Geometry: final body of the model. Coordinates: model frame, mm. A direction names the side the tool comes from. Round coordinates to 2 decimals unless told otherwise and drop trailing zeros. Loops run counter-clockwise (first coordinate to the right, second up) from the corner with the lowest first, then second, coordinate; pieces in that order, holes last. Notation, with made-up numbers: M 40.25,51.25 L 89.25,51.25 A23 ccw 89.25,74.25 Z; hole C -21.5,26 d8. An arc over 180 degrees is marked long. Write each question's results on one line, items separated by ' | '.
```python
from build123d import *

# Parameters (mm, degrees)
BOX018_W               = 0.3
BOX018_H               = 3.5
BOX018_DEPTH           = 4
BOX018_PLACEMENT_ANGLE = 120
BOX017_W               = 0.3
BOX017_H               = 3.5
BOX017_DEPTH           = 4
BOX017_PLACEMENT_ANGLE = 120
BOX016_W               = 0.3
BOX016_H               = 3.5
BOX016_DEPTH           = 4
BOX016_PLACEMENT_ANGLE = 120
BOX014_W               = 0.3
BOX014_H               = 3.5
BOX014_DEPTH           = 4
BOX003_W               = 0.3
BOX003_H               = 3.5
BOX003_DEPTH           = 4
BOX003_PLACEMENT_ANGLE = 30
BOX001_W               = 0.3
BOX001_H               = 3.5
BOX001_DEPTH           = 4
BOX001_PLACEMENT_ANGLE = 30
BOX002_W               = 0.3
BOX002_H               = 3.5
BOX002_DEPTH           = 4
BOX015_W               = 0.3
BOX015_H               = 3.5
BOX015_DEPTH           = 4
BOX004_W               = 0.3
BOX004_H               = 3.5
BOX004_DEPTH           = 4
BOX_W                  = 8
BOX_H                  = 4
BOX_DEPTH              = 4
CYLINDER001_R          = 2
CYLINDER001_DEPTH      = 4
CYLINDER_R             = 2
CYLINDER_DEPTH         = 4


with BuildPart() as cube018:
    # Box018 → Box018 (new body)
    with BuildSketch(Plane.XY):
        with Locations((0.15, 1.75)):
            Rectangle(BOX018_W, BOX018_H)
    extrude(amount=BOX018_DEPTH)


with BuildPart() as cube018_1:
    # Box018 placement: moved
    add(cube018.part.moved(Location((7.892915, 0.015358, 0))).rotate(Axis((7.892915, 0.015358, 0), (0, 0, -1)), BOX018_PLACEMENT_ANGLE))


with BuildPart() as cube017:
    # Box017 → Box017 (new body)
    with BuildSketch(Plane.XY):
        with Locations((0.15, 1.75)):
            Rectangle(BOX017_W, BOX017_H)
    extrude(amount=BOX017_DEPTH)


with BuildPart() as cube017_1:
    # Box017 placement: moved
    add(cube017.part.moved(Location((10.852236, 1.891667, 0))).rotate(Axis((10.852236, 1.891667, 0), (0, 0, 1)), BOX017_PLACEMENT_ANGLE))


with BuildPart() as cube016:
    # Box016 → Box016 (new body)
    with BuildSketch(Plane.XY):
        with Locations((0.15, 1.75)):
            Rectangle(BOX016_W, BOX016_H)
    extrude(amount=BOX016_DEPTH)


with BuildPart() as cube016_1:
    # Box016 placement: moved
    add(cube016.part.moved(Location((-0.004428, -0.104039, 0))).rotate(Axis((-0.004428, -0.104039, 0), (0, 0, 1)), BOX016_PLACEMENT_ANGLE))


with BuildPart() as cube014:
    # Box014 → Box014 (new body)
    with BuildSketch(Plane(origin=(2.3, 0, 0), x_dir=(1, 0, 0), z_dir=(0, 0, 1))):
        with Locations((0.15, 1.75)):
            Rectangle(BOX014_W, BOX014_H)
    extrude(amount=BOX014_DEPTH)


with BuildPart() as cube003:
    # Box003 → Box003 (new body)
    with BuildSketch(Plane.XY):
        with Locations((0.15, 1.75)):
            Rectangle(BOX003_W, BOX003_H)
    extrude(amount=BOX003_DEPTH)


with BuildPart() as cube003_1:
    # Box003 placement: moved
    add(cube003.part.moved(Location((7.7321, -3, 0))).rotate(Axis((7.7321, -3, 0), (0, 0, 1)), BOX003_PLACEMENT_ANGLE))


with BuildPart() as cube001:
    # Box001 → Box001 (new body)
    with BuildSketch(Plane.XY):
        with Locations((0.15, 1.75)):
            Rectangle(BOX001_W, BOX001_H)
    extrude(amount=BOX001_DEPTH)


with BuildPart() as cube001_1:
    # Box001 placement: moved
    add(cube001.part.rotate(Axis((0, 0, 0), (0, 0, 1)), BOX001_PLACEMENT_ANGLE))


with BuildPart() as cube002:
    # Box002 → Box002 (new body)
    with BuildSketch(Plane(origin=(6, 0, 0), x_dir=(1, 0, 0), z_dir=(0, 0, 1))):
        with Locations((0.15, 1.75)):
            Rectangle(BOX002_W, BOX002_H)
    extrude(amount=BOX002_DEPTH)


with BuildPart() as cube015:
    # Box015 → Box015 (new body)
    with BuildSketch(Plane(origin=(3.6, -3.5, 0), x_dir=(1, 0, 0), z_dir=(0, 0, 1))):
        with Locations((0.15, 1.75)):
            Rectangle(BOX015_W, BOX015_H)
    extrude(amount=BOX015_DEPTH)


with BuildPart() as fusion008:
    # Box004 → Box004 (new body)
    with BuildSketch(Plane(origin=(0, -3.5, 0), x_dir=(1, 0, 0), z_dir=(0, 0, 1))):
        with Locations((0.15, 1.75)):
            Rectangle(BOX004_W, BOX004_H)
    extrude(amount=BOX004_DEPTH)

    # Fusion008: union Cube018, Cube017, Cube016, Cube014, Cube003, Cube001, Cube002, Cube015
    add(cube018_1.part)
    add(cube017_1.part)
    add(cube016_1.part)
    add(cube014.part)
    add(cube003_1.part)
    add(cube001_1.part)
    add(cube002.part)
    add(cube015.part)


with BuildPart() as cube:
    # Box → Box (new body)
    with BuildSketch(Plane(origin=(0, -2, 0), x_dir=(1, 0, 0), z_dir=(0, 0, 1))):
        with Locations((4, 2)):
            Rectangle(BOX_W, BOX_H)
    extrude(amount=BOX_DEPTH)


with BuildPart() as cylinder001:
    # Cylinder001 → Cylinder001 (new body)
    with BuildSketch(Plane(origin=(8, 0, 0), x_dir=(1, 0, 0), z_dir=(0, 0, 1))):
        Circle(CYLINDER001_R)
    extrude(amount=CYLINDER001_DEPTH)


with BuildPart() as fusion014:
    # Cylinder → Cylinder (new body)
    with BuildSketch(Plane.XY):
        Circle(CYLINDER_R)
    extrude(amount=CYLINDER_DEPTH)

    # Fusion: union Cube, Cylinder001
    add(cube.part)
    add(cylinder001.part)

    # Fusion014: union Fusion008
    add(fusion008.part)


solid = fusion014.part
```
1. Ray query, probe 1 along Y at (x, z) = (1.75, 1.85); probe 2 along Y at (x, z) = (2.5, 0.85); probe 3 along X at (y, z) = (-1.25, 1.1). Return the intervals inside material, ascending.
Answer key:
probe 1: y = -2 to 2 | probe 2: y = -2 to 3.5 | probe 3: x = -2.59 to -1.99, -1.56 to 10.08
2. Pin query (flat end, axial travel): P1, Ø0.8, axis at y = 3, z = 2, coming from the +X side; P2, Ø0.8, axis at y = 3, z = 2.5, coming from the -X side; P3, Ø1.5, axis at x = 7.5, z = 1.5, coming from the -Y side. Return the tip coordinate at first contact, or that it passes through.
Answer key:
P1: stops at x = 6.3 | P2: stops at x = -1.75 | P3: stops at y = -3
3. Draft query along Y for faces 4 (the face through (2.3, 3, 2)), 5 (the face through (1, 2, 2)), 6 (the face through (7.75, -2.43, 1.97)). Return one class per face: pulls with the +Y half, pulls with the -Y half, needs draft (parallel to the pull), parting line crosses it, or undercut.
Answer key:
face 4: needs draft | face 5: pulls with the +Y half | face 6: undercut
4. Access query for faces 1 (the face through (-1.37, 2.37, 1.97)), 2 (the face through (10.069, 1.786, 1.972)), 3 (the face through (10.147, -1.632, 1.972)). Directions: +Z, -Z, +X, -X, +Y, -Y. A direction counts if a zero-diameter tool reaches every point of the face in a straight line with its end or side. Return the directions, or none.
Answer key:
face 1: +Z, -Z, -X | face 2: +Z, -Z, +Y | face 3: +Z, -Z, -Y
5. Section C-C (y = 0.75). Output: boundary loops of the cut face in (x, z).
Answer key:
outline: M -1.85,0 L 9.85,0 L 9.85,4 L -1.85,4 Z
6. Section A-A (y = 2.75). Output: boundary loops of the cut face in (x, z), then the cut area to 3 significant figures.
Answer key:
outline: M -1.59,0 L -1.24,0 L -1.24,4 L -1.59,4 Z; M 2.3,0 L 2.6,0 L 2.6,4 L 2.3,4 Z; M 6,0 L 6.3,0 L 6.3,4 L 6,4 Z | area: 3.79 mm²
7. Section B-B (x = 4.25). Output: boundary loops of the cut face in (y, z).
Answer key:
outline: M -2,0 L 2,0 L 2,4 L -2,4 Z
